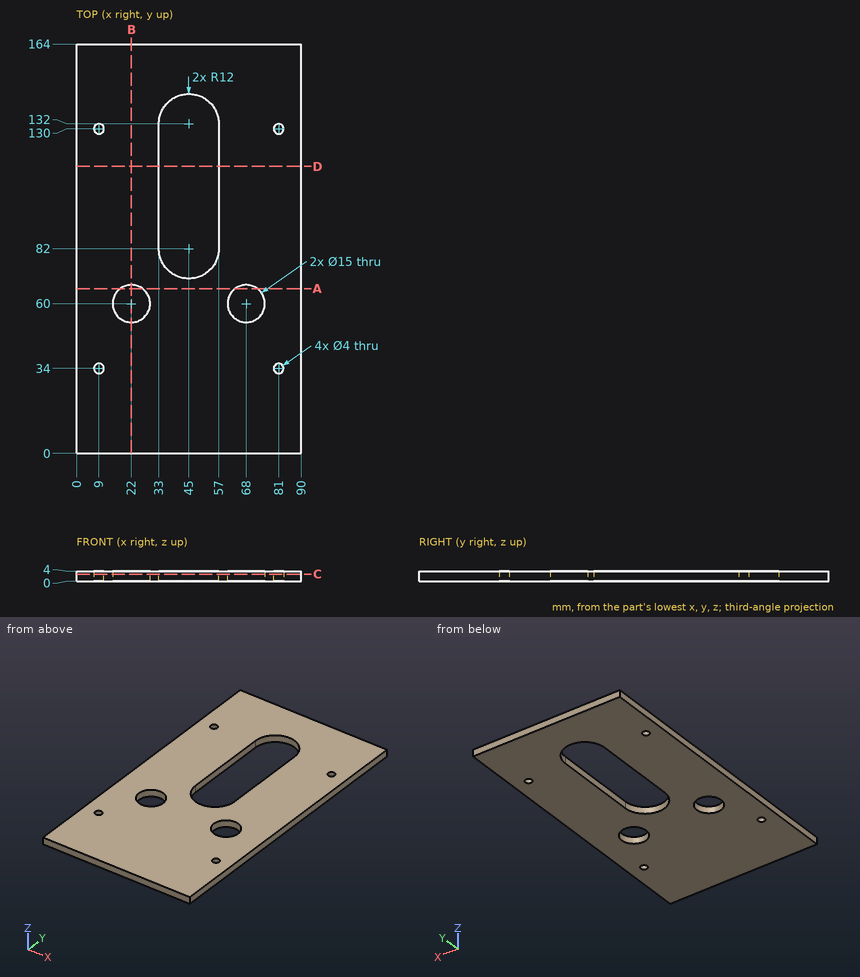
Verification items for this drawing (mm, ordinates from the low corner). Give positions to 0.01 mm unless a question says otherwise; leave off trailing zeros. Loops run counter-clockwise (first coordinate to the right, second up) from the corner with the lowest first, then second, coordinate; pieces in that order, holes last. Notation, with made-up numbers: M 46,69.5 L 70,69.5 A15 ccw 70,89.5 Z; hole C 21.5,58.5 d3. An arc over 180 degrees is marked long. Answer as a JSON object with one key per item and string values. Group by question number.
Item 1: Sectioned sample at D-D on y = 115. Record the boundary of the cut face in (x, z), plus the area to 3 significant figures.
Item 2: Sectioned sample at C-C on z = 2.9. Record the boundary of the cut face in (x, y).
Item 3: Material ranges on L1, parallel to Y at x = 81, z = 1; L2, parallel to X at y = 130, z = 1.05; L3, parallel to X at y = 118, z = 3.5, recorded low to high.
Item 4: Sectioned sample at A-A on y = 66. Record the boundary of the cut face in (x, z), plus the area to 3 significant figures.
Item 5: Sectioned sample at B-B on x = 22. Record the boundary of the cut face in (y, z), plus the area to 3 significant figures.
Findings below:
{
 "1": {"outline": "M 0,0 L 33,0 L 33,4 L 0,4 Z; M 57,0 L 90,0 L 90,4 L 57,4 Z", "area": "264 mm2"},
 "2": {"outline": "M 0,0 L 90,0 L 90,164 L 0,164 Z; hole C 9,34 d4; hole C 9,130 d4; hole C 22,60 d15; hole M 33,82 A12 ccw 57,82 L 57,132 A12 ccw 33,132 Z; hole C 68,60 d15; hole C 81,34 d4; hole C 81,130 d4"},
 "3": {"L1": "0 to 32, 36 to 128, 132 to 164", "L2": "0 to 7, 11 to 33, 57 to 79, 83 to 90", "L3": "0 to 33, 57 to 90"},
 "4": {"outline": "M 0,0 L 17.5,0 L 17.5,4 L 0,4 Z; M 26.5,0 L 63.5,0 L 63.5,4 L 26.5,4 Z; M 72.5,0 L 90,0 L 90,4 L 72.5,4 Z", "area": "288 mm2"},
 "5": {"outline": "M 0,0 L 52.5,0 L 52.5,4 L 0,4 Z; M 67.5,0 L 164,0 L 164,4 L 67.5,4 Z", "area": "596 mm2"}
}
